Autodesk Inventor part; units mm, degrees
ref_plane "Work Plane1" through (-173.9561, 20, -439.4442) normal (0, 1, 0) x (1, 0, 0)
ref_plane "Work Plane2" through (-173.9561, 5, -439.4442) normal (0, -1, 0) x (1, 0, 0)
ref_plane "YZ Plane" through (0, 0, 0) normal (1, 0, 0) x (0, 1, 0)
sketch "Sketch1" plane through (0, 0, 0) normal (0, 1, 0) x (-1, 0, 0)
  circle A0 centre (173.9561, -439.4442) radius 14
  dimension "d17" = 28
extrude "Extrusion1" add sketch "Sketch1" against normal blind 10
sketch "Sketch2" plane through (-173.9561, -10, -439.4442) normal (0, -1, 0) x (1, 0, 0)
  circle A0 centre (0, 0) radius 15.25
  point P0 (173.9561, 439.4442)
  dimension "d20" = 30.5
extrude "Extrusion2" add sketch "Sketch2" along normal blind 12
chamfer "Chamfer1" distance 1.25 angle 45 1 edges at (-189.2061, -10, -439.4442)
sketch "Sketch4" plane through (-173.9561, -22, -439.4442) normal (0, -1, 0) x (1, 0, 0)
  circle A0 centre (0, 0) radius 14
  point P0 (173.9561, 439.4442)
  dimension "d26" = 28
extrude "Extrusion3" add sketch "Sketch4" along normal blind 0.5
sketch "Sketch5" plane through (-173.9561, -22.5, -439.4442) normal (0, -1, 0) x (1, 0, 0)
  circle A0 centre (0, 0) radius 15.25
  point P0 (173.9561, 439.4442)
  dimension "d29" = 30.5
extrude "Extrusion4" add sketch "Sketch5" along normal blind 28
sketch "Sketch6" plane through (-173.9561, -50.5, -439.4442) normal (0, -1, 0) x (1, 0, 0)
  circle A0 centre (0, 0) radius 14
  point P0 (173.9561, 439.4442)
  dimension "d32" = 28
extrude "Extrusion5" add sketch "Sketch6" along normal blind 5
sketch "Sketch7" plane through (-173.9561, 0, -439.4442) normal (0, 1, 0) x (1, 0, 0)
  circle A0 centre (0, 0) radius 15.25
  point P0 (173.9561, -439.4442)
  dimension "d35" = 30.5
extrude "Extrusion6" add sketch "Sketch7" along normal blind 30
sketch "Sketch8" plane through (-173.9561, 30, -439.4442) normal (0, 1, 0) x (1, 0, 0)
  circle A0 centre (0, 0) radius 9
  point P0 (173.9561, -439.4442)
  dimension "d38" = 18
extrude "Extrusion7" add sketch "Sketch8" along normal blind 3
sketch "Sketch10" plane through (-173.9561, 33, -439.4442) normal (0, 1, 0) x (1, 0, 0)
  circle A0 centre (0, 0) radius 6.0592
  point P0 (173.9561, -439.4442)
extrude "Extrusion9" add sketch "Sketch10" along normal blind 2
sketch "Sketch11" plane through (-173.9561, 35, -439.4442) normal (0, 1, 0) x (1, 0, 0)
  circle A0 centre (0, 0) radius 2
  point P0 (173.9561, -439.4442)
  dimension "d45" = 4
extrude "Extrusion10" add sketch "Sketch11" along normal blind 16
fillet "Fillet1" radius 0.5 1 edges at (-175.9561, 51, -439.4442)
sketch "Sketch12" plane through (-173.9561, 51, -439.4442) normal (0, 1, 0) x (1, 0, 0)
  circle A0 centre (0, 0) radius 2
  circle A1 centre (0, 0) radius 2
  line L0 (-1.75, -0.9682) -> (-1.75, 0.9682)
  line L1 (1.75, -0.9682) -> (1.75, 0.9682)
  point P0 (173.9561, -439.4442)
  dimension "d49" = 3.5
  dimension "d50" = 1.75
extrude "Extrusion11" cut sketch "Sketch12" against normal blind 14 contours A0 L1 | L0 A0
ref_plane "Work Plane1" through (-173.9561, 20, -439.4442) normal (0, 1, 0) x (1, 0, 0)
ref_plane "Work Plane2" through (-173.9561, 5, -439.4442) normal (0, -1, 0) x (1, 0, 0)
split_face "Split1"
split_face "Split2"
equation "\"d50\" = 0.5 * d49"
properties part number "14-0009"
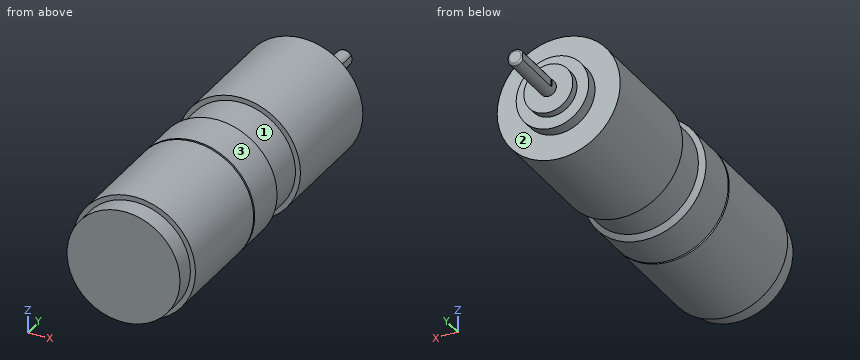
Input: part model. Units: mm. Frame: model coordinates. Face numbers are marked on the shaded views. A direction names the side the tool comes from. Give positions to 0.01 mm unless a question says otherwise; leave off trailing zeros. Order: outer loops, then holes, each group sorted by start corner. A loop starts at its lowest first (then second) coordinate and runs counter-clockwise, first axis right, second up.
Q1. Section B-B on y = 43. Output: boundary loops of the cut face in (x, z), and give its area (3 significant figures).
Checked values:
outline: (-175.71, -440.41) arc R2 ccw to (-172.21, -440.41) - (-172.21, -438.48) arc R2 ccw to (-175.71, -438.48) - close
area: 11.9 mm2
Q2. Section A-A on y = -9. Output: boundary loops of the cut face in (x, z).
Checked values:
outline: circle Ø28 at (-173.96, -439.44)
Q3. Section C-C on y = -37. Output: boundary loops of the cut face in (x, z), and give its area (3 significant figures).
Checked values:
outline: circle Ø30.5 at (-173.96, -439.44)
area: 731 mm2
Q4. Contact query for flat-ended pins moving along their axis: pin 1 Ø6 at (x, y) = (-184.5, -21.5) entering from +Z; pin 2 Ø2 at (y, z) = (44.5, -439.5) entering from -X; pin 3 Ø8.5 at (x, z) = (-178, -445) entering from +Y. Output: stop coordinate, or through.
Checked values:
pin 1: stops at z = -426.19
pin 2: stops at x = -175.71
pin 3: stops at y = 35
Q5. Set-up query: the marked faces 1, 2 and 3. Return all of +Z, -Z, +X, -X, +Y, -Y with unobstructed straight access to the full face (end or side cutting, diameter ignored); none if empty.
Checked values:
face 1: none
face 2: +Y
face 3: +Y, -Y
Q6. Ray query, probe 1 along Y at (x, z) = (-181, -452); probe 2 along Y at (x, z) = (-162.5, -433.5); probe 3 along Y at (x, z) = (-166, -437.5). Return the intervals inside material, ascending.
Checked values:
probe 1: y = -50.5 to -22.5, -22 to -10.4, 0 to 30
probe 2: y = -55.5 to 30
probe 3: y = -55.5 to 33
